Geometry check sheet. Reference: the model listing, model coordinates, mm. A direction names the side the tool comes from. Give positions to 0.01 mm unless a question says otherwise; leave off trailing zeros. Loops run counter-clockwise (first coordinate to the right, second up) from the corner with the lowest first, then second, coordinate; pieces in that order, holes last. Notation, with made-up numbers: (38, 11.5) -> (55, 11.5) arc R11 cw to (55, 18.5) -> close; hole circle Ø2 at (5, 35). An arc over 180 degrees is marked (long way). Write item = value, one per line.
```python
from build123d import *

# Parameters (mm, degrees)
SKETCH_1_R      = 1.6
EXTRUDE_1_DEPTH = 2
FILLET_1_R      = 20


with BuildPart() as part:
    # ｽｹｯﾁ1 → ﾎﾞｽ - 押し出し1 (new body)
    with BuildSketch(Plane.XY):
        with BuildLine():
            ThreePointArc((87, 38.5), (90.5, 35), (87, 31.5))
            Line((87, 31.5), (58.272014636, 31.5))
            Line((58.272014636, 31.5), (48.343911087, 48.69597977))
            ThreePointArc((48.343911087, 48.69597977), (49.625, 53.477068684), (54.406088913, 52.19597977))
            Line((54.406088913, 52.19597977), (62.313466521, 38.5))
            Line((62.313466521, 38.5), (87, 38.5))
        make_face()
        with Locations((87, 35)):
            Circle(SKETCH_1_R, mode=Mode.SUBTRACT)
        with Locations((75, 35)):
            Circle(SKETCH_1_R, mode=Mode.SUBTRACT)
        with Locations((55.375, 43.51777654)):
            Circle(SKETCH_1_R, mode=Mode.SUBTRACT)
        with Locations((51.375, 50.44597977)):
            Circle(SKETCH_1_R, mode=Mode.SUBTRACT)
    extrude(amount=EXTRUDE_1_DEPTH)

    # ﾌｨﾚｯﾄ1
    fillet_1_edges = [part.edges().sort_by_distance(p)[0] for p in [
        (58.272014636, 31.5, 1),
        (62.313466521, 38.5, 1),
    ]]
    fillet(fillet_1_edges, radius=FILLET_1_R)


solid = part.part
```
Item 1: Tool access check on faces 5 (the flat face through (80, 38.5, 1)), 6 (the cylindrical face through (76.48, 34.39, 0.99)). Record the directions out of +Z, -Z, +X, -X, +Y, -Y that give a thin tool (end or side, any length) a straight path to the whole face; none if there is none.
Answer:
face_5 = +Z, -Z, +X, +Y
face_6 = +Z, -Z
Item 2: Section check C-C, the plane y = 35. Record the cut outline in (x, z).
Answer:
outline = (58.52, 0) -> (73.4, 0) -> (73.4, 2) -> (58.52, 2) -> close; (76.6, 0) -> (85.4, 0) -> (85.4, 2) -> (76.6, 2) -> close; (88.6, 0) -> (90.5, 0) -> (90.5, 2) -> (88.6, 2) -> close
Item 3: Thickness scan on L1, parallel to Y at x = 87, z = 0.55; L2, parallel to X at y = 34.75, z = 1.55; L3, parallel to Y at x = 79.5, z = 1.9. Record the ranges inside material, lowest first. Write a range as [from, to].
Answer:
L1 = [31.5, 33.4], [36.6, 38.5]
L2 = [58.89, 73.42], [76.58, 85.42], [88.58, 90.49]
L3 = [31.5, 38.5]
Item 4: Section check A-A, the plane x = 75. Record the cut outline in (y, z), plus the area to 3 significant figures.
Answer:
outline = (31.5, 0) -> (33.4, 0) -> (33.4, 2) -> (31.5, 2) -> close; (36.6, 0) -> (38.5, 0) -> (38.5, 2) -> (36.6, 2) -> close
area = 7.60 mm^2
Item 5: Gauge pin test, flat ends, axial feed: pin 1 (0.6 mm diameter, centred on x = 83.5, z = 1, fed in from +Y); pin 2 (1.9 mm diameter, centred on x = 55.38, y = 43.52, fed in from +Z); pin 3 (1 mm diameter, centred on y = 36, z = 0, fed in from -X). Record the tip position at first contact, or that the pin passes through.
Answer:
pin_1 = 38.5
pin_2 = through
pin_3 = 56.59
Item 6: Section check B-B, the plane y = 49.75. Record the cut outline in (x, z), plus the area to 3 significant figures.
Answer:
outline = (47.94, 0) -> (49.93, 0) -> (49.93, 2) -> (47.94, 2) -> close; (52.82, 0) -> (55.82, 0) -> (55.82, 2) -> (52.82, 2) -> close
area = 9.98 mm^2
Item 7: Section check D-D, the plane z = 1.4. Record the cut outline in (x, y) (3 decimals).
Answer:
outline = (48.344, 48.696) -> (52.499, 41.5) arc R20 ccw to (69.819, 31.5) -> (87, 31.5) arc R3.5 ccw to (87, 38.5) -> (73.86, 38.5) arc R20 cw to (56.54, 48.5) -> (54.406, 52.196) arc R3.5 ccw to start; hole circle Ø3.2 at (51.375, 50.446); hole circle Ø3.2 at (55.375, 43.518); hole circle Ø3.2 at (75, 35); hole circle Ø3.2 at (87, 35)
Item 8: Draft check along Y on faces 1 (the cylindrical face through (85.73, 34.03, 0.99)), 2 (the cylindrical face through (64, 41.1, 1)), 3 (the cylindrical face through (59.946, 34.107, 1.014)), 4 (the cylindrical face through (56.235, 44.867, 0.986)). Enter one of: +Y half, -Y half, draft (parallel to the pull), parting line (faces both ways), or undercut.
Answer:
face_1 = undercut
face_2 = +Y half
face_3 = -Y half
face_4 = undercut
